Geometry check sheet. Reference: the model listing, model coordinates, mm. Face numbers are marked on the shaded views. A direction names the side the tool comes from. Round coordinates to 2 decimals unless told otherwise and drop trailing zeros. Loops run counter-clockwise (first coordinate to the right, second up) from the corner with the lowest first, then second, coordinate; pieces in that order, holes last. Notation, with made-up numbers: (59.5, 60.25) -> (84.5, 60.25) arc R31 cw to (84.5, 91.25) -> close; hole circle Ø8 at (-30, 63). An arc over 180 degrees is marked (long way). Use a Markdown table: item, result. Add a question column.
Q1. Set-up check for the marked faces 1 and 2: record each of +Z, -Z, +X, -X, +Y, -Y from which the full face is reachable in a straight line by a thin tool's end or side.
Q2. Gauge pin test, flat end, axial feed: P1, Ø1.5, axis at x = 15, z = -10, coming from the +Y side. Record the tip position at first contact, or that the pin passes through.
Q3. Sectioned sample at A-A, the plane y = -2.35. Enter the section's corners in (x, z), then the cut area to 3 significant figures.
Q4. Sectioned sample at D-D, the plane z = -10. Enter the section's corners in (x, y) (3 decimals), then the cut area to 3 significant figures.
Q5. Sectioned sample at B-B, the plane z = 0. Enter the section's corners in (x, y) (3 decimals).
Q6. Release check for a two-part mould opening along Z. For the marked faces 3, 4 and 5 record: released by +Z, released by -Z, zero draft, split by the parting line, or undercut.
Q7. Sectioned sample at C-C, the plane x = 9.5. Enter the section's corners in (y, z) (3 decimals).
Q8. Material ranges on L1, parallel to Z at x = -9, y = -2.8; L2, parallel to Z at x = 10.5, y = -2.85; L3, parallel to X at y = -2.15, z = -1.25, recorded low to high.
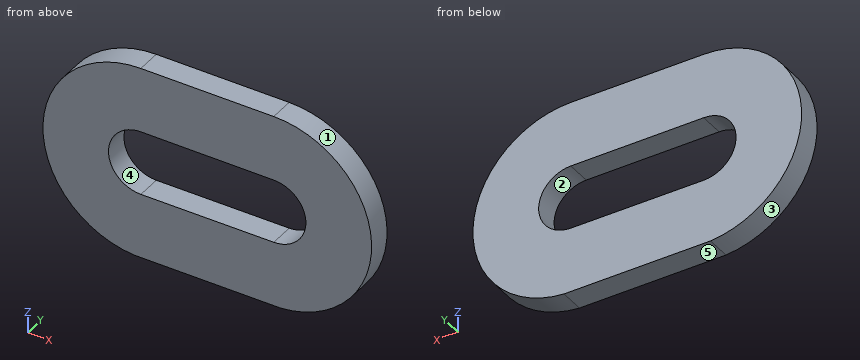
```python
from build123d import *

# Parameters (mm, degrees)
F1_DEPTH = 3.175


with BuildPart() as f1:
    # F0 (on Front) → F1 (new body)
    with BuildSketch(Plane.XZ):
        with BuildLine():
            Line((-9.992783, -12.638227), (8.961562, -12.638227))
            ThreePointArc((8.961562, -12.638227), (20.74528, 0.439046), (8.084128, 12.668776))
            Line((8.084128, 12.668776), (-9.114507, 12.668711))
            ThreePointArc((-9.114507, 12.668711), (-21.775548, 0.439403), (-9.992783, -12.638227))
        make_face()
        with BuildLine():
            ThreePointArc((-9.108698, -4.185383), (-13.299846, -1.6e-05), (-9.108729, 4.185383))
            Line((-9.108729, 4.185383), (8.089874, 4.161838))
            ThreePointArc((8.089874, 4.161838), (12.245952, 8.1e-05), (8.089905, -4.161707))
            Line((8.089905, -4.161707), (-9.108698, -4.185383))
        make_face(mode=Mode.SUBTRACT)
    extrude(amount=F1_DEPTH)


solid = f1.part
```
Values:
| question | item | result |
|---|---|---|
| 1 | face 1 | +X, +Y, -Y |
| 1 | face 2 | +Y, -Y |
| 2 | P1 | y = 0 |
| 3 | outline | (-9.99, -12.64) -> (8.96, -12.64) arc R12.67 ccw to (8.08, 12.67) -> (-9.11, 12.67) arc R12.67 ccw to start; hole (-9.11, -4.19) -> (8.09, -4.16) arc R4.16 ccw to (8.09, 4.16) -> (-9.11, 4.19) arc R4.19 ccw to start |
| 3 | area | 741 mm^2 |
| 4 | outline | (-16.892, -3.175) -> (15.862, -3.175) -> (15.862, 0) -> (-16.892, 0) -> close |
| 4 | area | 104 mm^2 |
| 5 | outline | (-21.783, -3.175) -> (-13.3, -3.175) -> (-13.3, 0) -> (-21.783, 0) -> close; (12.246, -3.175) -> (20.753, -3.175) -> (20.753, 0) -> (12.246, 0) -> close |
| 6 | face 3 | split by the parting line |
| 6 | face 4 | undercut |
| 6 | face 5 | released by -Z |
| 7 | outline | (-3.175, -12.589) -> (0, -12.589) -> (0, -3.913) -> (-3.175, -3.913) -> close; (-3.175, 3.914) -> (0, 3.914) -> (0, 12.589) -> (-3.175, 12.589) -> close |
| 8 | L1 | -12.64 to -4.19, 4.19 to 12.67 |
| 8 | L2 | -12.44 to -3.39, 3.39 to 12.44 |
| 8 | L3 | -21.72 to -13.11, 12.05 to 20.69 |
